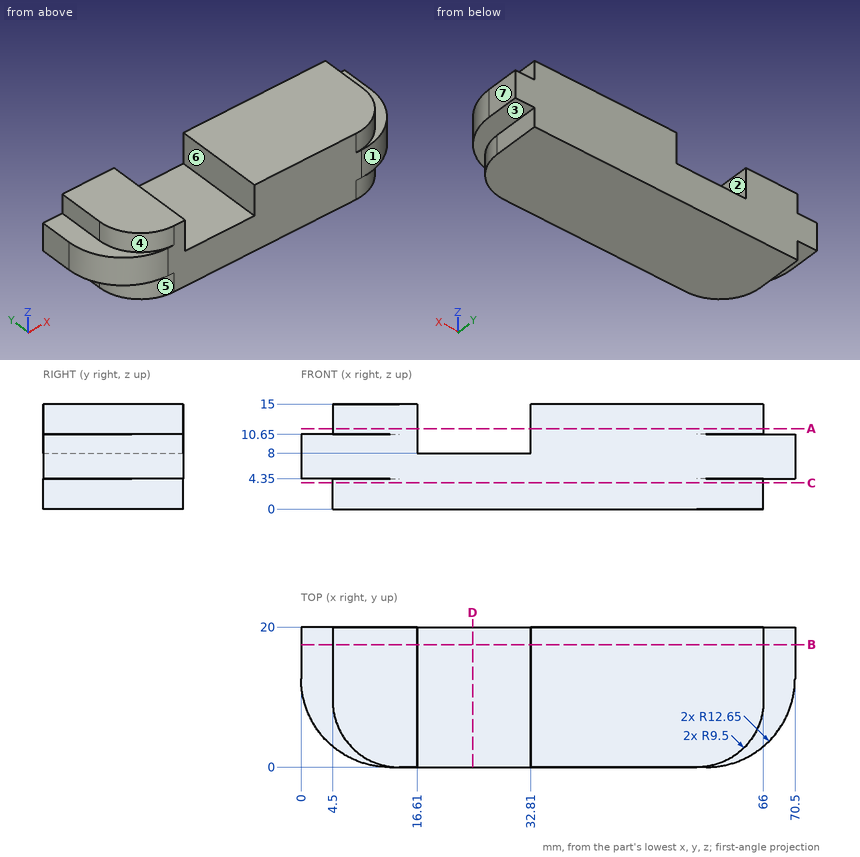
Design review of the part shown in the three views and the two pictorial views. Dimensions are in mm from the part's minimum x, y and z. A direction names the side the tool comes from. Coordinates: 2 decimals unless noted, no trailing zeros. Loops run counter-clockwise (first coordinate to the right, second up) from the corner with the lowest first, then second, coordinate; pieces in that order, holes last.
Q1. Tool access review of the marked faces 4, 5, 6 and 7: name each direction out of +Z, -Z, +X, -X, +Y, -Y from which nothing blocks a thin tool from reaching the whole face with its end or side.
Reported:
face 4: +Z, -X, -Y
face 5: -Z, -X, -Y
face 6: +Z, +Y, -Y
face 7: +Z, -Z, +X, +Y, -Y
Q2. We need section D-D on x = 24.5. State the section outline as (y, z) points, and give its area (3 significant figures).
Reported:
outline: (0, 0) - (20, 0) - (20, 8) - (0, 8) - close
area: 160 mm2
Q3. We need section A-A on z = 11.5. State the section outline as (x, y) points, and give its area (3 significant figures).
Reported:
outline: (4.5, 9.5) arc R9.5 ccw to (14, 0) - (16.61, 0) - (16.61, 20) - (4.5, 20) - close; (32.81, 0) - (56.5, 0) arc R9.5 ccw to (66, 9.5) - (66, 20) - (32.81, 20) - close
area: 867 mm2
Q4. We need section C-C on z = 3.75. State the section outline as (x, y) points.
Reported:
outline: (4.5, 9.5) arc R9.5 ccw to (14, 0) - (56.5, 0) arc R9.5 ccw to (66, 9.5) - (66, 20) - (4.5, 20) - close
Q5. The part is to be moulded in two halves that separate along X. For the marked faces 1, 2 and 3, say which applies: +X half, -X half, draft (parallel to the pull), parting line (faces both ways), or undercut.
Reported:
face 1: +X half
face 2: undercut
face 3: draft
Q6. To check wall thickness, follow line 1 (X direction, y = 12, z = 14); line 2 (Z direction, x = 29, y = 5.25); line 3 (X direction, y = 1, z = 10.75). State the ranges of each line that lie inside material, in increasing order.
Reported:
line 1: x = 4.5 to 16.61, 32.81 to 66
line 2: z = 0 to 8
line 3: x = 9.76 to 16.61, 32.81 to 60.74
Q7. For pin 1 (5 mm diameter, centred on y = 16.5, z = 12.5, fed in from +X); pin 2 (10 mm diameter, centred on x = 27.5, y = 2.5, fed in from +Z); pin 3 (3.5 mm diameter, centred on y = 15, z = 1.5, fed in from +X); pin 4 (7.5 mm diameter, centred on y = 6.5, z = 12, fed in from -X), all flat-tipped, find the tip position at first contact; note any pin that passes through.
Reported:
pin 1: stops at x = 70.5
pin 2: stops at z = 8
pin 3: stops at x = 66
pin 4: stops at x = 0.28
Q8. We need section B-B on y = 17.5. State the section outline as (x, z) points.
Reported:
outline: (0, 4.35) - (4.5, 4.35) - (4.5, 0) - (66, 0) - (66, 4.35) - (70.5, 4.35) - (70.5, 10.65) - (66, 10.65) - (66, 15) - (32.81, 15) - (32.81, 8) - (16.61, 8) - (16.61, 15) - (4.5, 15) - (4.5, 10.65) - (0, 10.65) - close
